Autodesk Inventor part; units mm, degrees
ref_plane "YZ Plane" through (0, 0, 0) normal (1, 0, 0) x (0, 1, 0)
ref_plane "XZ Plane" through (0, 0, 0) normal (0, 1, 0) x (-1, 0, 0)
ref_plane "XY Plane" through (0, 0, 0) normal (0, 0, 1) x (1, 0, 0)
sketch "Sketch7" plane through (0, 0, 0) normal (1, 0, 0) x (0, 1, 0)
  line L0 (4.585, 16.5) -> (-4.585, 16.5)
  line L1 (-4.585, 16.5) -> (-4.585, -16.5)
  line L2 (-4.585, -16.5) -> (4.585, -16.5)
  line L3 (4.585, -16.5) -> (4.585, 16.5)
  circle A0 centre (0, 14.3) radius 1.25
  circle A1 centre (0, -14.3) radius 1.25
  line L4 (4.585, 0) -> (-4.585, 0) construction
  line L5 (4.585, 11.585) -> (-4.585, 11.585)
  line L6 (4.585, -11.585) -> (-4.585, -11.585)
  point P0 (0, 0)
  point P1 (0, 16.5)
  point P2 (0, 0)
  dimension "d85" = 33
  dimension "d86" = 9.17
  dimension "d87" = 2.5
  dimension "d89" = 28.6
  dimension "d90" = 23.17
extrude "Extrusion3" add sketch "Sketch7" along normal blind 3
fillet "Fillet1" radius 2 1 edges at (1.5, 4.585, 16.5)
fillet "Fillet2" radius 2 1 edges at (1.5, 4.585, -16.5)
fillet "Fillet3" radius 2 1 edges at (1.5, -4.585, -16.5)
fillet "Fillet4" radius 2 1 edges at (1.5, -4.585, 16.5)
sketch "Sketch8" plane through (3, 0, 0) normal (1, 0, 0) x (0, 0, -1)
  line L0 (14.5, 4.585) -> (-14.5, 4.585)
  line L1 (-14.5, -4.585) -> (14.5, -4.585)
  line L2 (-11.585, 4.585) -> (11.585, 4.585)
  line L3 (11.585, 4.585) -> (11.585, -4.585)
  line L4 (11.585, -4.585) -> (-11.585, -4.585)
  line L5 (-11.585, -4.585) -> (-11.585, 4.585)
  line L6 (0, 4.585) -> (0, -4.585) construction
  line L7 (-11.585, 4.585) -> (11.585, 4.585)
  line L8 (11.585, -4.585) -> (-11.585, -4.585)
  point P0 (0, 0)
  point P1 (0, 0)
  point P2 (0, 4.585)
  point P3 (-11.585, -4.585)
  point P4 (11.585, 4.585)
  dimension "d97" = 23.17
extrude "Extrusion4" add sketch "Sketch8" along normal blind 7 and the other way blind 17.05
sketch "Sketch9" plane through (10, 0, 0) normal (1, 0, 0) x (0, 0, -1)
  circle A0 centre (-4, 0) radius 2.5
  point P0 (0, 0)
  dimension "d102" = 5
  dimension "d103" = 4
extrude "Extrusion5" add sketch "Sketch9" along normal blind 4
sketch "Sketch11" plane through (14, 0, 4) normal (1, 0, 0) x (0, 0, -1)
  circle A0 centre (0, 0) radius 1.25
  circle A1 centre (0, 0) radius 2.5
  point P0 (4, 0)
  dimension "d107" = 2.5
extrude "Extrusion6" cut sketch "Sketch11" against normal blind 7 contours A0
properties part number "6P-014"
Can you work these out from the model? Positions are in its coordinate system, mm. A direction names the side the tool comes from. Give positions to 0.01 mm unless a question says otherwise; leave off trailing zeros. Loops run counter-clockwise (first coordinate to the right, second up) from the corner with the lowest first, then second, coordinate; pieces in that order, holes last. Notation, with made-up numbers: (38, 66) - (82, 66) arc R23 ccw to (82, 103) - close; hole circle Ø11 at (37, -36.5). An arc over 180 degrees is marked (long way). One line per item, written item: value.
(1) If we section it at D-D, the plane y = 3: List the corners of the cut face in (x, z) for me (3 decimals).
Verdict:
outline: (-14.05, -11.585) - (0, -11.585) - (0, -16.456) - (3, -16.456) - (3, -11.585) - (10, -11.585) - (10, 11.585) - (3, 11.585) - (3, 16.456) - (0, 16.456) - (0, 11.585) - (-14.05, 11.585) - close
(2) I'm going to push flat-ended pins straight in: pin 1 (3 mm diameter, centred on x = -7, y = 0.5, fed in from +Z) (3 decimals); pin 2 (4 mm diameter, centred on y = 1, z = -14, fed in from +X); pin 3 (2 mm diameter, centred on y = -0.5, z = -8, fed in from +X); pin 4 (2 mm diameter, centred on y = 0.5, z = 4.5, fed in from +X). Where does each tip first touch, or does it pass through?
Verdict:
pin 1: z = 11.585
pin 2: x = 3
pin 3: x = 10
pin 4: x = 14
(3) If we section it at B-B, the plane x = 7.75: List the corners of the cut face in (y, z) for me (3 decimals).
Verdict:
outline: (-4.585, -11.585) - (4.585, -11.585) - (4.585, 11.585) - (-4.585, 11.585) - close; hole circle Ø2.5 at (0, 4)
(4) On a 3-axis mill with a long thin cutter (end or side, diameter ignored), from which of +Z, -Z, +X, -X, +Y, -Y can I reach the whole of each face in a straight line? I mean faces 1 (the face through (0, -1, 13)), 2 (the face through (11.972, -0.751, 1.615)), 3 (the face through (0, -0.1, -12.9)). Say none if no direction works.
Verdict:
face 1: +Z, -X, +Y, -Y
face 2: +X
face 3: -Z, -X, +Y, -Y
(5) I need wall thicknesses on line 1 along Z through (x, y) = (2.05, 0); line 2 along X through (y, z) = (-1.75, -8.5); line 3 along Y through (x, z) = (8.5, 4) (3 decimals). Which ranges of each line are inside material? Lowest first, please.
Verdict:
line 1: -16.5 to -15.55, -13.05 to 13.05, 15.55 to 16.5
line 2: -14.05 to 10
line 3: -4.585 to -1.25, 1.25 to 4.585
(6) If we section it at C-C, the plane z = 4: List the corners of the cut face in (x, y) for me (3 decimals).
Verdict:
outline: (-14.05, -4.585) - (10, -4.585) - (10, -2.5) - (14, -2.5) - (14, -1.25) - (7, -1.25) - (7, 1.25) - (14, 1.25) - (14, 2.5) - (10, 2.5) - (10, 4.585) - (-14.05, 4.585) - close
(7) If we section it at A-A, the plane y = -0.75: List the corners of the cut face in (x, z) for me (3 decimals).
Verdict:
outline: (-14.05, -11.585) - (0, -11.585) - (0, -13.3) - (3, -13.3) - (3, -11.585) - (10, -11.585) - (10, 1.615) - (14, 1.615) - (14, 3) - (7, 3) - (7, 5) - (14, 5) - (14, 6.385) - (10, 6.385) - (10, 11.585) - (3, 11.585) - (3, 13.3) - (0, 13.3) - (0, 11.585) - (-14.05, 11.585) - close; (0, -16.5) - (3, -16.5) - (3, -15.3) - (0, -15.3) - close; (0, 15.3) - (3, 15.3) - (3, 16.5) - (0, 16.5) - close
(8) If we mould it in two halves opening along Z, with no side actions, what happens to faces 4 (the face through (-2, -4.585, 0)), 5 (the face through (7, 0, 4)), 6 (the face through (1.48, -0.16, 13.06)), 7 (the face through (6, 0, 11.585))? For each: released by +Z, released by -Z, zero draft, split by the parting line, or undercut.
Verdict:
face 4: zero draft
face 5: undercut
face 6: undercut
face 7: released by +Z
